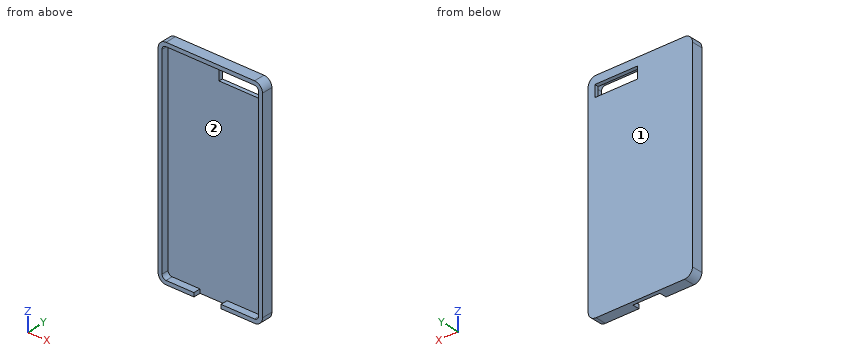
```python
from build123d import *

# Parameters (mm, degrees)
F0_W     = 67.1
F0_H     = 138.3
F1_DEPTH = 3.55
F2_R     = 5.08
F3_T     = -2.5
F4_W     = 27.54098
F4_H     = 7.459015
F5_DEPTH = 12.5
F6_W     = 17.408122
F6_H     = 4.6
F7_DEPTH = 25


with BuildPart() as f1:
    # F0 (on Front) → F1 (new body, symmetric)
    with BuildSketch(Plane.XZ):
        Rectangle(F0_W, F0_H)
    extrude(amount=F1_DEPTH, both=True)

    # F2
    f2_edges = [f1.edges().sort_by_distance(p)[0] for p in [
        (-33.55, 0, 69.15),
        (-33.55, 0, -69.15),
        (33.55, 0, -69.15),
        (33.55, 0, 69.15),
    ]]
    fillet(f2_edges, radius=F2_R)

    # F3
    f3_openings = [f1.faces().sort_by_distance(p)[0] for p in [
        (0, -3.55, 0),
    ]]
    offset(amount=F3_T, openings=f3_openings)

    # F4 (on Front) → F5 (cut, symmetric)
    with BuildSketch(Plane.XZ):
        with Locations((15.491805, 60.389347)):
            Rectangle(F4_W, F4_H)
    extrude(amount=F5_DEPTH, both=True, mode=Mode.SUBTRACT)

    # F6 (on face) → F7 (cut)
    with BuildSketch(Plane.XY.offset(-66.65)):
        with Locations((-1.833738, -1.25)):
            Rectangle(F6_W, F6_H)
    extrude(amount=-F7_DEPTH, mode=Mode.SUBTRACT)


solid = f1.part
```
Work out the finished part from the listing and answer in its coordinate system (mm). Face numbers are marked on the shaded views. Coordinates: 2 decimals unless noted, no trailing zeros. Write each loop counter-clockwise with the first axis right and the second up, starting at its lowest first coordinate (ties: lowest second). Pieces come first, ordered by that corner, then holes.
Q1. Determine the mould class of the marked faces 1 and 2 for opening direction Z: released by +Z, released by -Z, zero draft, split by the parting line, or undercut.
Q2. A cutting plane is placed at D-D, the plane y = -2. Give the vertices of the cut face in (x, z), then the cut area to 3 significant figures.
Q3. A cutting plane is placed at A-A, the plane x = 26.5. Give the vertices of the cut face in (y, z), then the cut area to 3 significant figures.
Q4. A cutting plane is placed at B-B, the plane z = 58.5. Give the vertices of the cut face in (x, y), then the cut area to 3 significant figures.
Q5. Find the intervals of material crossed by line 1 (X direction, y = -1, z = -58.5); line 2 (Z direction, x = 21, y = -0.75); line 3 (Z direction, x = 24, y = 2.5), in increasing order.
Q6. A cutting plane is placed at C-C, the plane z = -26. Give the vertices of the cut face in (x, y).
Q7. Each of these flat-tipped pins is pushed along its axis until it touches: pin 1 Ø2 at (y, z) = (-1.5, -68.5) entering from -X; pin 2 Ø1.5 at (x, z) = (-5.5, -20.5) entering from -Y; pin 3 Ø2 at (y, z) = (-1, -67.5) entering from +X. Where does it stop, or does it pass through?
Findings below:
1. face 1: zero draft
1. face 2: undercut
2. outline: (-33.55, -64.07) arc R5.08 ccw to (-28.47, -69.15) - (-10.54, -69.15) - (-10.54, -66.65) - (-28.47, -66.65) arc R2.58 cw to (-31.05, -64.07) - (-31.05, 64.07) arc R2.58 cw to (-28.47, 66.65) - (28.47, 66.65) arc R2.58 cw to (31.05, 64.07) - (31.05, -64.07) arc R2.58 cw to (28.47, -66.65) - (6.87, -66.65) - (6.87, -69.15) - (28.47, -69.15) arc R5.08 ccw to (33.55, -64.07) - (33.55, 64.07) arc R5.08 ccw to (28.47, 69.15) - (-28.47, 69.15) arc R5.08 ccw to (-33.55, 64.07) - close
2. area: 942 mm2
3. outline: (-3.55, -69.15) - (3.55, -69.15) - (3.55, 56.66) - (1.05, 56.66) - (1.05, -66.65) - (-3.55, -66.65) - close; (-3.55, 66.65) - (1.05, 66.65) - (1.05, 64.12) - (3.55, 64.12) - (3.55, 69.15) - (-3.55, 69.15) - close
3. area: 350 mm2
4. outline: (-33.55, -3.55) - (-31.05, -3.55) - (-31.05, 1.05) - (1.72, 1.05) - (1.72, 3.55) - (-33.55, 3.55) - close; (29.26, 1.05) - (31.05, 1.05) - (31.05, -3.55) - (33.55, -3.55) - (33.55, 3.55) - (29.26, 3.55) - close
4. area: 122 mm2
5. line 1: x = -33.55 to -31.05, 31.05 to 33.55
5. line 2: z = -69.15 to -66.65, 66.65 to 69.15
5. line 3: z = -69.15 to 56.66, 64.12 to 69.15
6. outline: (-33.55, -3.55) - (-31.05, -3.55) - (-31.05, 1.05) - (31.05, 1.05) - (31.05, -3.55) - (33.55, -3.55) - (33.55, 3.55) - (-33.55, 3.55) - close
7. pin 1: stops at x = -32.22
7. pin 2: stops at y = 1.05
7. pin 3: stops at x = 32.93
